Read the model definition and answer for the solid it produces. Units are mm, in the model's axes. Face numbers are marked on the shaded views. Give positions to 0.01 mm unless a question says otherwise; leave off trailing zeros. Order: outer loops, then holes, each group sorted by start corner. A loop starts at its lowest first (then second) coordinate and runs counter-clockwise, first axis right, second up. Notation, with made-up numbers: (37.5, -22) - (80.5, -22) arc R23 ccw to (80.5, 5) - close; hole circle Ø2 at (89, 34.5). An arc over 180 degrees is marked (long way). Use a Markdown table: item, result. Add a question column.
1. A cutting plane is placed at B-B on x = -266.7. Determine the outline of the cut face in (y, z), and give its area (3 significant figures).
2. A cutting plane is placed at C-C on y = -11.5. Determine the outline of the cut face in (x, z).
3. Consider L1, parallel to Z at x = 431.8, y = 2.25; L2, parallel to X at y = 2, z = 292; L3, parallel to Z at x = -266.7, y = 4.5. Determine where each line is inside the solid, lowest interval first.
4. A cutting plane is placed at D-D on z = 177.8. Determine the outline of the cut face in (x, y).
5. Flat-ended cylindrical pins translate along their axes: P1, Ø1.5, axis at x = -15, y = -19.5, coming from the +Z side; P2, Ø12.5, axis at y = -13.5, z = -38, coming from the +X side; P3, Ø4, axis at x = 187.5, z = -108.5, coming from the -Y side; P4, Ø23, axis at x = 190.5, z = 0, coming from the +Y side. Find the tip coordinate at first contact, or state that the pin passes through.
6. For a pull along Z with two mould halves and no side action, classify the marked faces 1 and 2 as released by +Z, released by -Z, zero draft, split by the parting line, or undercut.
7. A cutting plane is placed at A-A on z = 0. Determine the outline of the cut face in (x, y), and give its area (3 significant figures).
```python
from build123d import *

# Parameters (mm, degrees)
F0_W      = 990.6
F0_H      = 711.2
F1_DEPTH  = 9.017
F2_R      = 50.8
F3_R      = 3.96875
F4_DEPTH  = 9.018
F5_R      = 12.7
F6_DEPTH  = 9.018
F7_W      = 838.2
F7_H      = 558.8
F7_W_2    = 787.4
F7_H_2    = 508
F8_DEPTH  = 25.4
F9_R      = 57.15
F10_DEPTH = 9.018


with BuildPart() as f1:
    # F0 (on Front) → F1 (new body)
    with BuildSketch(Plane.XZ):
        Rectangle(F0_W, F0_H)
    extrude(amount=-F1_DEPTH)

    # F2
    f2_edges = [f1.edges().sort_by_distance(p)[0] for p in [
        (495.3, 4.5085, 355.6),
        (495.3, 4.5085, -355.6),
        (-495.3, 4.5085, -355.6),
        (-495.3, 4.5085, 355.6),
    ]]
    fillet(f2_edges, radius=F2_R)

    # F3 (on Front) → F4 (cut, through all)
    with BuildSketch(Plane.XZ):
        with Locations((-431.8, 292.1)):
            Circle(F3_R)
        with Locations((431.8, 292.1)):
            Circle(F3_R)
        with Locations((431.8, -292.1)):
            Circle(F3_R)
        with Locations((-431.8, -292.1)):
            Circle(F3_R)
    extrude(amount=-F4_DEPTH, mode=Mode.SUBTRACT)

    # F5 (on Front) → F6 (cut, through all)
    with BuildSketch(Plane.XZ):
        with Locations((190.5, 0)):
            Circle(F5_R)
    extrude(amount=-F6_DEPTH, mode=Mode.SUBTRACT)

    # F7 (on Front) → F8 (join)
    with BuildSketch(Plane.XZ):
        Rectangle(F7_W, F7_H)
        Rectangle(F7_W_2, F7_H_2, mode=Mode.SUBTRACT)
    extrude(amount=F8_DEPTH)

    # F9 (on Front) → F10 (cut, through all)
    with BuildSketch(Plane.XZ):
        with Locations((-266.7, 177.8)):
            Circle(F9_R)
        with Locations((-266.7, -177.8)):
            Circle(F9_R)
    extrude(amount=-F10_DEPTH, mode=Mode.SUBTRACT)


solid = f1.part
```
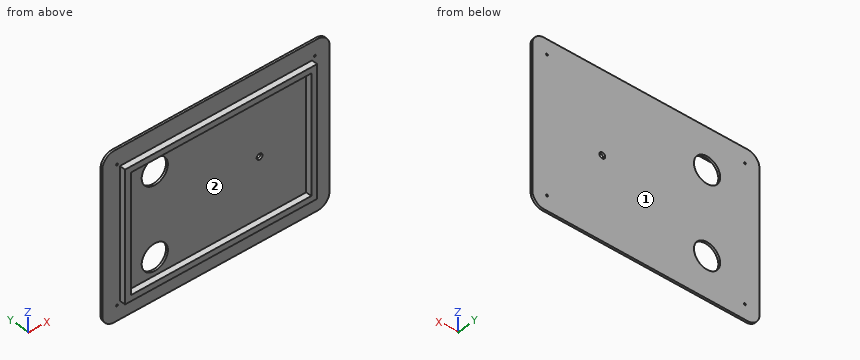
Output values:
| question | item | result |
|---|---|---|
| 1 | outline | (-25.4, -279.4) - (0, -279.4) - (0, -355.6) - (9.02, -355.6) - (9.02, -234.95) - (0, -234.95) - (0, -254) - (-25.4, -254) - close; (-25.4, 254) - (0, 254) - (0, 234.95) - (9.02, 234.95) - (9.02, 355.6) - (0, 355.6) - (0, 279.4) - (-25.4, 279.4) - close; (0, -120.65) - (9.02, -120.65) - (9.02, 120.65) - (0, 120.65) - close |
| 1 | area | 5,640 mm² |
| 2 | outline | (-419.1, -279.4) - (419.1, -279.4) - (419.1, 279.4) - (-419.1, 279.4) - close; hole (-393.7, -254) - (393.7, -254) - (393.7, 254) - (-393.7, 254) - close |
| 3 | L1 | -355.6 to -296.07, -288.13 to 288.13, 296.07 to 355.6 |
| 3 | L2 | -495.3 to -435.77, -427.83 to 427.83, 435.77 to 495.3 |
| 3 | L3 | -355.6 to -234.95, -120.65 to 120.65, 234.95 to 355.6 |
| 4 | outline | (-495.3, 0) - (-419.1, 0) - (-419.1, -25.4) - (-393.7, -25.4) - (-393.7, 0) - (-323.85, 0) - (-323.85, 9.02) - (-495.3, 9.02) - close; (-209.55, 0) - (393.7, 0) - (393.7, -25.4) - (419.1, -25.4) - (419.1, 0) - (495.3, 0) - (495.3, 9.02) - (-209.55, 9.02) - close |
| 5 | P1 | z = 279.4 |
| 5 | P2 | x = 419.1 |
| 5 | P3 | y = 0 |
| 5 | P4 | through |
| 6 | face 1 | zero draft |
| 6 | face 2 | undercut |
| 7 | outline | (-495.3, 0) - (-419.1, 0) - (-419.1, -25.4) - (-393.7, -25.4) - (-393.7, 0) - (177.8, 0) - (177.8, 9.02) - (-495.3, 9.02) - close; (203.2, 0) - (393.7, 0) - (393.7, -25.4) - (419.1, -25.4) - (419.1, 0) - (495.3, 0) - (495.3, 9.02) - (203.2, 9.02) - close |
| 7 | area | 9,990 mm² |
